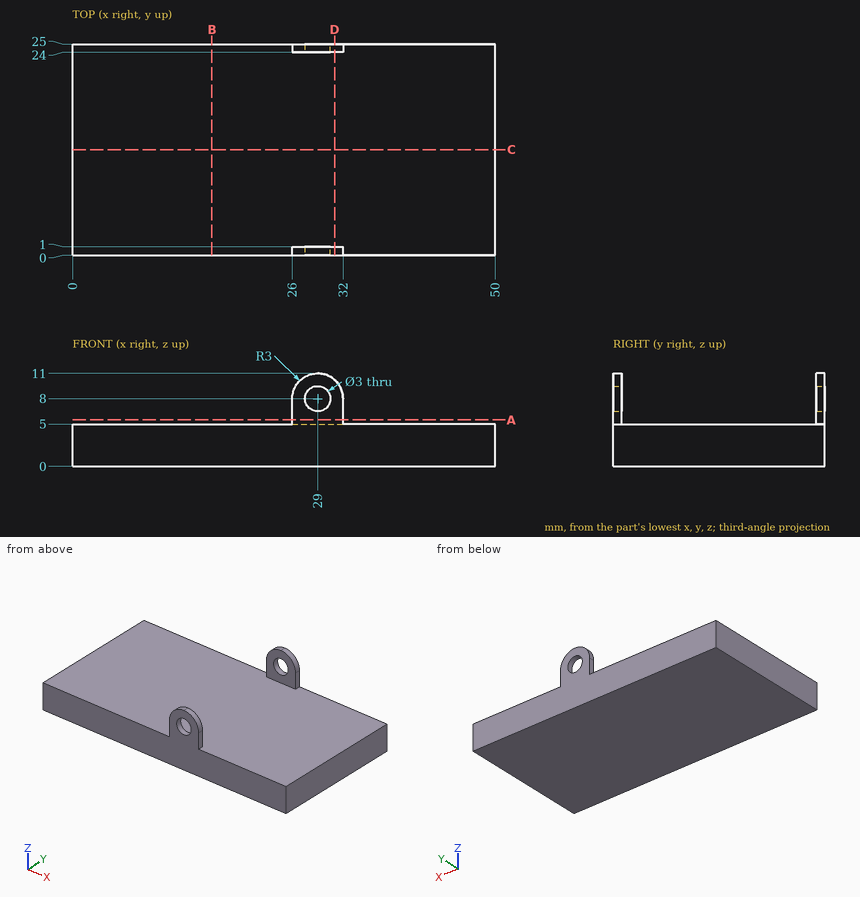
The figure shows three views and two pictorial views of one solid part (mm, origin at its lowest corner). Answer the questions. Round coordinates to 2 decimals unless told otherwise and drop trailing zeros. Write each loop counter-clockwise with the first axis right and the second up, starting at its lowest first coordinate (ties: lowest second). Pieces come first, ordered by that corner, then holes. Notation, with made-up numbers: M -20,-25 L 13,-25 A18 cw 13,7 Z; hole C -11.5,55.25 d1. An arc over 180 degrees is marked long. Use a Markdown table: item, result.
1) Straight lines are drawn through the part: line 1 along Z through (x, y) = (29, 24.75); line 2 along Z through (x, y) = (8, 10.5). For each, find the intervals that lie inside material, in ascending order. Write a range as [from, to].
Answers follow:
| item | result |
|---|---|
| line 1 | z = [0, 6.5], [9.5, 11] |
| line 2 | z = [0, 5] |
2) Flat-ended cylindrical pins translate along their axes: pin 1 (4 mm diameter, centred on y = 12, z = 7.5, fed in from +X); pin 2 (0.8 mm diameter, centred on y = 0.5, z = 6.5, fed in from +X); pin 3 (12.5 mm diameter, centred on x = 22, y = 10.5, fed in from +Z); pin 4 (0.8 mm diameter, centred on y = 0.5, z = 7, fed in from -X). Find the tip coordinate at first contact, or state that the pin passes through.
Answers follow:
| item | result |
|---|---|
| pin 1 | passes through |
| pin 2 | stops at x = 32 |
| pin 3 | stops at z = 5 |
| pin 4 | stops at x = 26 |
3) The part is cut by section B-B (x = 16.5). Write down the section's boundary in (y, z), plus the area to 3 significant figures.
Answers follow:
| item | result |
|---|---|
| outline | M 0,0 L 25,0 L 25,5 L 0,5 Z |
| area | 125 mm2 |
4) The part is cut by section A-A (z = 5.5). Write down the section's boundary in (x, y).
Answers follow:
| item | result |
|---|---|
| outline | M 26,0 L 32,0 L 32,1 L 26,1 Z; M 26,24 L 32,24 L 32,25 L 26,25 Z |
5) The part is cut by section D-D (x = 31). Write down the section's boundary in (y, z).
Answers follow:
| item | result |
|---|---|
| outline | M 0,0 L 25,0 L 25,10.24 L 24,10.24 L 24,5 L 1,5 L 1,10.24 L 0,10.24 Z |
6) The part is cut by section C-C (y = 12.5). Write down the section's boundary in (x, z).
Answers follow:
| item | result |
|---|---|
| outline | M 0,0 L 50,0 L 50,5 L 0,5 Z |
